For this review, take the finished solid that the model builds, in its own axes (mm). A direction names the side the tool comes from. Round coordinates to 2 decimals unless told otherwise and drop trailing zeros. Loops run counter-clockwise (first coordinate to the right, second up) from the corner with the lowest first, then second, coordinate; pieces in that order, holes last.
1) Take a section at A-A (y = 8). State the section outline as (x, z) points.
2) Take a section at C-C (z = 3.4). State the section outline as (x, y) points.
3) Tool access review of faces 4 (the flat face through (-9, -0.388, 1)), 5 (the flat face through (4, 3, 1.8)), 6 (the flat face through (12, 10, 1)): name each direction out of +Z, -Z, +X, -X, +Y, -Y from which nothing blocks a thin tool from reaching the whole face with its end or side.
4) Wall thickness on L1, parallel to X at y = 0.25, z = 1.95; L2, parallel to X at y = 9.25, z = 0.9; L3, parallel to Z at x = 12.5, y = 3: over which ranges is each line inside the solid? List them lowest first.
5) Mouldability with a two-part tool opening along Y and no side actions: class faces 1 (the cylindrical face through (7.868, -1.149, 0.913)), 2 (the flat face through (-1, 3, 0)), 3 (the cylindrical face through (14, -5, 1)) as pulls with the +Y half, pulls with the -Y half, needs draft (parallel to the pull), parting line crosses it, or undercut.
6) Take a section at B-B (x = -7). State the section outline as (y, z) points.
7) Take a section at D-D (x = 18). State the section outline as (y, z) points, then the cut area to 3 significant figures.
8) Insertion check: pin 1 (1.4 mm diameter, centred on x = 24, z = 1, fed in from +Y); pin 2 (2 mm diameter, centred on y = 10, z = 1, fed in from +X); pin 3 (0.5 mm diameter, centred on x = -17.5, z = 1.5, fed in from -Y); pin 4 (5 mm diameter, centred on x = 5.1, y = 0, fed in from +Z). Each pin has a flat end and moves straight along its axis. Give the tip position at first contact, or say it passes through.
```python
from build123d import *

# Parameters (mm, degrees)
F0_W        = 18.7768550515
F0_H        = 8
F0_W_2      = 1.2231449485
F1_DEPTH    = 1.8
F2_R        = 3
F2_R_2      = 1.5
F3_DEPTH    = 1.801
F4_W        = 3
F4_H        = 8
F5_DEPTH    = 3
F6_R        = 5
F7_T1_DEPTH = 1.8


# Not quite as in the source:
# - a fillet or chamfer that OpenCascade refuses, or shapes differently, is made with other operations: its cross-section is extruded or revolved along the edge and cut away or added


with BuildPart() as f1:
    # F0 (on Top) → F1 (new body)
    with BuildSketch(Plane.XY):
        with BuildLine():
            ThreePointArc((-1.1898192428, -11.2838109608), (0.0506537792, -11.8176267396), (1.3887392017, -12))
            Line((1.3887392017, -12), (12, -12))
            Line((12, -12), (12, -4))
            Line((12, -4), (10.7768550515, -4))
            Line((10.7768550515, -4), (10.7768550515, 4))
            Line((10.7768550515, 4), (12, 4))
            Line((12, 4), (12, 12))
            Line((12, 12), (1.3906232978, 12))
            ThreePointArc((1.3906232978, 12), (0.0508527618, 11.8171583855), (-1.1909314511, 11.2820059643))
            Line((-1.1909314511, 11.2820059643), (-19.9959281202, 2.3695112828))
            Line((-19.9959281202, 2.3695112828), (-17.9959281202, 0.3695112828))
            Line((-17.9959281202, 0.3695112828), (-16.4537748835, 0.3695112828))
            ThreePointArc((-16.4537748835, 0.3695112828), (-15, 1.5), (-13.5462251165, 0.3695112828))
            Line((-13.5462251165, 0.3695112828), (-4.2914064974, 0.3695112828))
            Line((-4.2914064974, 0.3695112828), (-4.2914064974, -0.3879051656))
            Line((-4.2914064974, -0.3879051656), (-13.5510246439, -0.3879051656))
            ThreePointArc((-13.5510246439, -0.3879051656), (-15, -1.5), (-16.4489753561, -0.3879051656))
            Line((-16.4489753561, -0.3879051656), (-17.9941705506, -0.3879051656))
            Line((-17.9941705506, -0.3879051656), (-19.9941705506, -2.3879051656))
            Line((-19.9941705506, -2.3879051656), (-1.1898192428, -11.2838109608))
        make_face()
        with Locations((21.3884275258, 0)):
            Rectangle(F0_W, F0_H)
        with Locations((11.3884275258, 0)):
            Rectangle(F0_W_2, F0_H)
    extrude(amount=F1_DEPTH)

    # F2 (on face) → F3 (cut, through all)
    with BuildSketch(Plane.XY.offset(1.8)):
        with Locations((5.0964765251, 8)):
            Circle(F2_R)
        with Locations((5.0964765251, 0)):
            Circle(F2_R)
        with Locations((5.0964765251, -8)):
            Circle(F2_R)
        with Locations((-1.1856243946, 0)):
            Circle(F2_R_2)
    extrude(amount=-F3_DEPTH, mode=Mode.SUBTRACT)

    # F4 (on face) → F5 (join)
    with BuildSketch(Plane.XY.offset(1.8)):
        with Locations((29.2768550515, 0)):
            Rectangle(F4_W, F4_H)
    extrude(amount=F5_DEPTH)

    # F6
    f6_edges = [f1.edges().sort_by_distance(p)[0] for p in [
        (12, 4, 0.9),
        (12, -4, 0.9),
    ]]
    fillet(f6_edges, radius=F6_R)

    # F7: fillet of radius 0.5 on 2 edges, made by hand

    # F7_s2 → F7_t1 (join)
    with BuildSketch(Plane.XY):
        with BuildLine():
            ThreePointArc((-4.2914064974, 0.1120948344), (-4.4378531068, -0.2414585561), (-4.7914064974, -0.3879051656))
            Line((-4.7914064974, -0.3879051656), (-4.2914064974, -0.3879051656))
            Line((-4.2914064974, -0.3879051656), (-4.2914064974, 0.1120948344))
        make_face()
        with BuildLine():
            ThreePointArc((-4.7914064974, 0.3695112828), (-4.4378531068, 0.2230646734), (-4.2914064974, -0.1304887172))
            Line((-4.2914064974, -0.1304887172), (-4.2914064974, 0.3695112828))
            Line((-4.2914064974, 0.3695112828), (-4.7914064974, 0.3695112828))
        make_face()
    extrude(amount=F7_T1_DEPTH)


solid = f1.part
```
Response:
1. outline: (-8.12, 0) - (2.1, 0) - (2.1, 1.8) - (-8.12, 1.8) - close; (8.1, 0) - (12.1, 0) - (12.1, 1.8) - (8.1, 1.8) - close
2. outline: (27.78, -4) - (30.78, -4) - (30.78, 4) - (27.78, 4) - close
3. face 4: +Z, -Z, -X
3. face 5: +Z, -X, +Y, -Y
3. face 6: +Z, -Z, +X, +Y
4. L1: x = 27.78 to 30.78
4. L2: x = -5.48 to 2.37, 7.82 to 12
4. L3: z = 0 to 1.8
5. face 1: undercut
5. face 2: needs draft
5. face 3: pulls with the -Y half
6. outline: (-8.54, 0) - (-0.39, 0) - (-0.39, 1.8) - (-8.54, 1.8) - close; (0.37, 0) - (8.53, 0) - (8.53, 1.8) - (0.37, 1.8) - close
7. outline: (-4, 0) - (4, 0) - (4, 1.8) - (-4, 1.8) - close
7. area: 14.4 mm2
8. pin 1: stops at y = 4
8. pin 2: stops at x = 12
8. pin 3: stops at y = -3.69
8. pin 4: passes through
